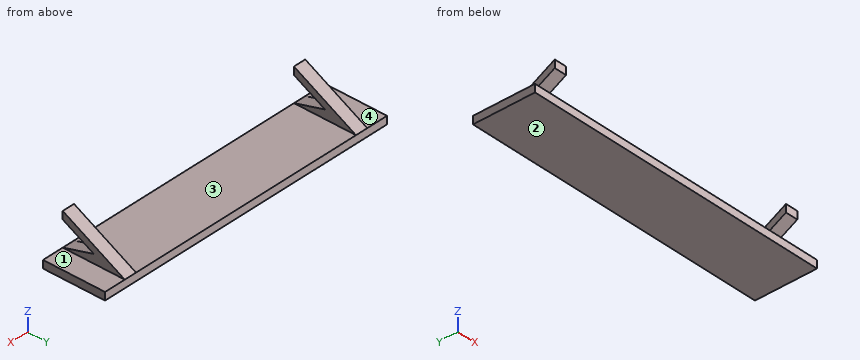
```python
from build123d import *

# Parameters (mm, degrees)
SKETCH_W     = 100
SKETCH_H     = 20
PAD_DEPTH    = 2.5
PAD001_DEPTH = 2


with BuildPart() as part:
    # Sketch → Pad (new body)
    with BuildSketch(Plane.XY):
        Rectangle(SKETCH_W, SKETCH_H)
    extrude(amount=PAD_DEPTH)

    # Sketch002 (on DatumPlane) → Pad001 (join, symmetric)
    with BuildSketch(Plane.YZ.offset(-41)):
        Polygon((10, 2.5), (-10, 13.134189), (-10, 10.634189), (0, 5.317094), (-10, 2.5), align=None)
    pad001 = extrude(amount=PAD001_DEPTH, both=True)

    # Mirrored: Pad001 across YZ
    add(pad001.mirror(Plane.YZ))


solid = part.part
```
Design review of the part built by this model. Coordinates are the model's own, in mm. Face numbers are marked on the shaded views. A direction names the side the tool comes from. Coordinates: 2 decimals unless noted, no trailing zeros. Loops run counter-clockwise (first coordinate to the right, second up) from the corner with the lowest first, then second, coordinate; pieces in that order, holes last.
Q1. We need section C-C on y = -5.75. State the section outline as (x, z) points, and give its area (3 significant figures).
Reported:
outline: (-50, 0) - (50, 0) - (50, 2.5) - (43, 2.5) - (43, 3.7) - (39, 3.7) - (39, 2.5) - (-39, 2.5) - (-39, 3.7) - (-43, 3.7) - (-43, 2.5) - (-50, 2.5) - close; (-43, 8.37) - (-39, 8.37) - (-39, 10.87) - (-43, 10.87) - close; (39, 8.37) - (43, 8.37) - (43, 10.87) - (39, 10.87) - close
area: 280 mm2
Q2. We need section B-B on z = 3.75. State the section outline as (x, y) points, and give its area (3 significant figures).
Reported:
outline: (-43, -5.56) - (-39, -5.56) - (-39, 7.65) - (-43, 7.65) - close; (39, -5.56) - (43, -5.56) - (43, 7.65) - (39, 7.65) - close
area: 106 mm2
Q3. We need section D-D on y = 5.75. State the section outline as (x, z) points, and give its area (3 significant figures).
Reported:
outline: (-50, 0) - (50, 0) - (50, 2.5) - (43, 2.5) - (43, 4.76) - (39, 4.76) - (39, 2.5) - (-39, 2.5) - (-39, 4.76) - (-43, 4.76) - (-43, 2.5) - (-50, 2.5) - close
area: 268 mm2
Q4. For pin 1 (4 mm diameter, centred on y = -5.5, z = 11.5, fed in from -X); pin 2 (12 mm diameter, centred on x = 36, y = 6.5, fed in from +Z); pin 3 (3.5 mm diameter, centred on x = -47.5, y = -2.5, fed in from +Z); pin 4 (1 mm diameter, centred on y = -1, z = 11, fed in from +X), all flat-tipped, find the tip position at first contact; note any pin that passes through.
Reported:
pin 1: stops at x = -43
pin 2: stops at z = 7.12
pin 3: stops at z = 2.5
pin 4: passes through
Q5. The part is to be moulded in two halves that separate along X. For the marked faces 3 and 4, say which applies: +X half, -X half, draft (parallel to the pull), parting line (faces both ways), or undercut.
Reported:
face 3: undercut
face 4: draft
Q6. To check wall thickness, follow line 1 (X direction, y = -6.5, z = 9.5); line 2 (Z direction, x = -30, y = -8.5). State the ranges of each line that lie inside material, in increasing order.
Reported:
line 1: x = -43 to -39, 39 to 43
line 2: z = 0 to 2.5
Q7. Tool access review of the marked faces 1 and 2: name each direction out of +Z, -Z, +X, -X, +Y, -Y from which nothing blocks a thin tool from reaching the whole face with its end or side.
Reported:
face 1: +Z, +X, +Y, -Y
face 2: -Z, +X, -X, +Y, -Y
Q8. We need section A-A on x = 41. State the section outline as (y, z) points.
Reported:
outline: (-10, 0) - (10, 0) - (10, 2.5) - (-10, 13.13) - (-10, 10.63) - (0, 5.32) - (-10, 2.5) - close
